Part print with two shaded views. Sizes in mm from the minimum x, y, z corner. A direction names the side the tool comes from. Coordinates: 2 decimals unless noted, no trailing zeros. Loops run counter-clockwise (first coordinate to the right, second up) from the corner with the lowest first, then second, coordinate; pieces in that order, holes last. Notation, with made-up numbers: (22, -27.5) - (66, -27.5) arc R21 ccw to (66, -20.5) - close; hole circle Ø6 at (9.5, -32). An arc over 180 degrees is marked (long way). Answer as CSV lines item,"result".
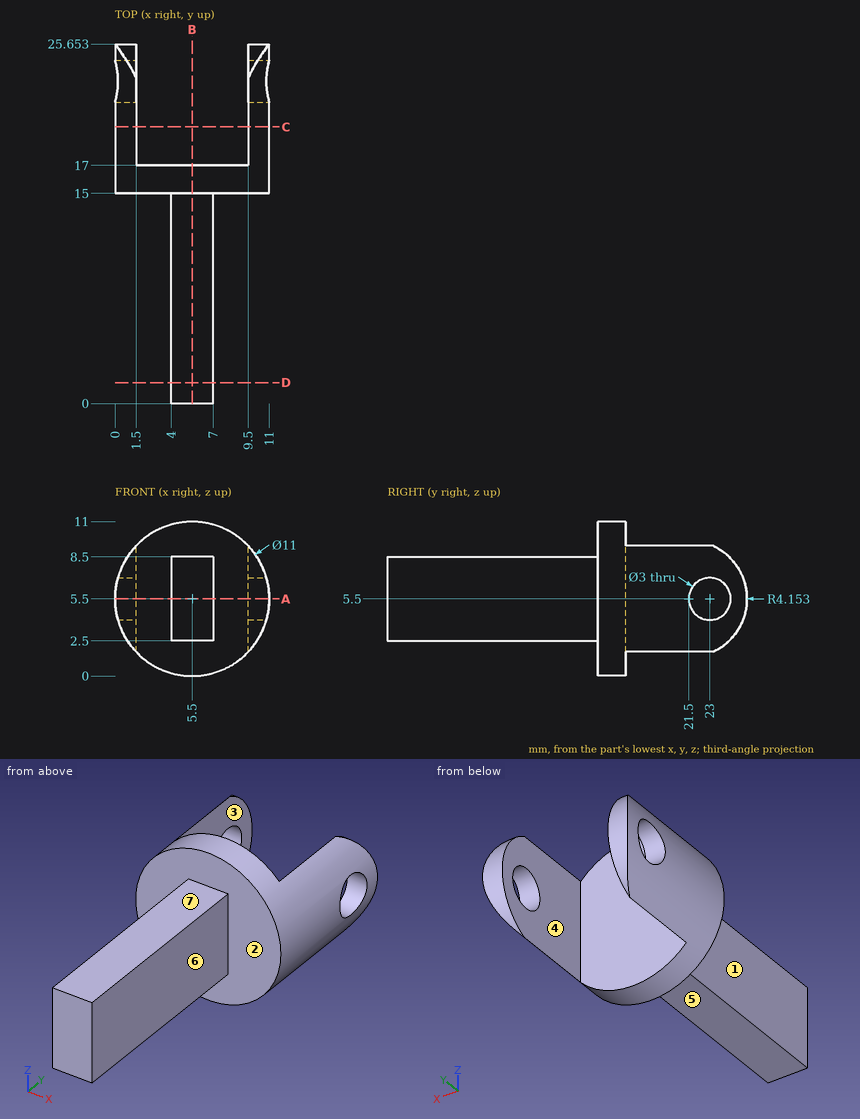
Q1. Saw through at A-A (z = 5.5). Give the cut face in (x, y).
Results:
outline,"(0, 15) - (4, 15) - (4, 0) - (7, 0) - (7, 15) - (11, 15) - (11, 21.5) - (9.5, 21.5) - (9.5, 17) - (1.5, 17) - (1.5, 21.5) - (0, 21.5) - close; (0, 24.5) - (1.5, 24.5) - (1.5, 25.65) - (0, 25.65) - close; (9.5, 24.5) - (11, 24.5) - (11, 25.65) - (9.5, 25.65) - close"
Q2. Two-plate mould, pull along X, no slides. Class the marked faces 1, 2 and 3: released by +X, released by -X, zero draft, split by the parting line, or undercut.
Results:
face 1,"released by -X"
face 2,"zero draft"
face 3,"undercut"
Q3. Saw through at C-C (y = 19.75). Give the cut face in (x, z) (1 decimal).
Results:
outline,"(1.5, 1.7) - (1.5, 9.3) arc R5.5 ccw to start; (9.5, 1.7) arc R5.5 ccw to (9.5, 9.3) - close"
Q4. Which spindle directions (+Z, -Z, +X, -X, +Y, -Y) get a long thin tool onto all of the face, cutting with end or side? Do the marked faces 4, 5, 6 and 7. Say none if no direction does.
Results:
face 4,"+Z, -Z, +Y"
face 5,"-Z, +X, -X, -Y"
face 6,"+Z, -Z, +X, -Y"
face 7,"+Z, +X, -X, -Y"
Q5. Wall check: L1, parallel to Y at x = 0.35, z = 5.5; L2, parallel to Y at x = 8, z = 8; L3, parallel to Z at x = 10.15, y = 23 (1 decimal). Give the ranges that are in metal, low to high.
Results:
L1,"y = 15 to 21.5, 24.5 to 25.65"
L2,"y = 15 to 17"
L3,"z = 2.6 to 4, 7 to 8.4"
Q6. Saw through at B-B (x = 5.5). Give the cut face in (y, z).
Results:
outline,"(0, 2.5) - (15, 2.5) - (15, 0) - (17, 0) - (17, 11) - (15, 11) - (15, 8.5) - (0, 8.5) - close"
Q7. Saw through at D-D (y = 1.5). Give the cut face in (x, z), then the cut area to 3 significant figures.
Results:
outline,"(4, 2.5) - (7, 2.5) - (7, 8.5) - (4, 8.5) - close"
area,"18.0 mm^2"
Q8. Flat gauge pins, fed straight in: pin 1 (2.5 mm diameter, centred on y = 23, z = 5.5, fed in from +X); pin 2 (5 mm diameter, centred on y = 8.5, z = 6, fed in from -X); pin 3 (3.5 mm diameter, centred on x = 5, y = 5, fed in from +Z); pin 4 (2.5 mm diameter, centred on x = 5.5, y = 10, fed in from -Z). Where does each tip first touch, or does it go through?
Results:
pin 1,"passes through"
pin 2,"stops at x = 4"
pin 3,"stops at z = 8.5"
pin 4,"stops at z = 2.5"
